from build123d import *

# Parameters (mm, degrees)
SKETCH1_W                    = 41
SKETCH1_H                    = 20
BASE_FLANGE1_DEPTH           = 0.7
EDGE_FLANGE1_STRIP_W         = 4.324
EDGE_FLANGE1_STRIP_H         = 0.7
EDGE_FLANGE1_STRIP_CUT_DEPTH = 20
EDGE_FLANGE1_DEPTH           = 20
EDGE_FLANGE2_STRIP_W         = 4.324
EDGE_FLANGE2_STRIP_H         = 0.7
EDGE_FLANGE2_STRIP_CUT_DEPTH = 20
EDGE_FLANGE2_DEPTH           = 20
M3_CLEARANCE_HOLE1_D         = 3.4


# Sheet-metal steps are written as plain solids
with BuildPart() as part:
    # Sketch1 → Base-Flange1 (new body)
    with BuildSketch(Plane(origin=(0, 0, 0), x_dir=(1, 0, 0), z_dir=(0, 1, 0))):
        with Locations((20.5, 10)):
            Rectangle(SKETCH1_W, SKETCH1_H)
    extrude(amount=-BASE_FLANGE1_DEPTH)

    # Edge-Flange1 strip (across the edge) → Edge-Flange1 strip cut (cut)
    with BuildSketch(Plane(origin=(41, 0, 0), x_dir=(-1, 0, 0), z_dir=(0, 0, -1))):
        with Locations((-1.4, -0.35)):
            Rectangle(EDGE_FLANGE1_STRIP_W, EDGE_FLANGE1_STRIP_H)
    edge_flange1_strip_cut = extrude(amount=EDGE_FLANGE1_STRIP_CUT_DEPTH, mode=Mode.SUBTRACT)

    # Edge-Flange1 section (across the edge) → Edge-Flange1 (add)
    with BuildSketch(Plane(origin=(41, 0, 0), x_dir=(-1, 0, 0), z_dir=(0, 0, -1))):
        with BuildLine():
            Line((-0.7, 0.762), (-0.7, 20.25))
            Line((-0.7, 20.25), (0, 20.25))
            Line((0, 20.25), (0, 0.762))
            ThreePointArc((0, 0.762), (0.223184633, 0.223184633), (0.762, 0))
            Line((0.762, 0), (0.762, -0.7))
            ThreePointArc((0.762, -0.7), (-0.271790114, -0.271790114), (-0.7, 0.762))
        make_face()
    edge_flange1 = extrude(amount=EDGE_FLANGE1_DEPTH)

    # Edge-Flange2 strip (across the edge) → Edge-Flange2 strip cut (cut)
    with BuildSketch(Plane(origin=(41.7, 20.25, -20), x_dir=(0, -1, 0), z_dir=(0, 0, 1))):
        with Locations((-0.7, -0.35)):
            Rectangle(EDGE_FLANGE2_STRIP_W, EDGE_FLANGE2_STRIP_H)
    edge_flange2_strip_cut = extrude(amount=EDGE_FLANGE2_STRIP_CUT_DEPTH, mode=Mode.SUBTRACT)

    # Edge-Flange2 section (across the edge) → Edge-Flange2 (add)
    with BuildSketch(Plane(origin=(41.7, 20.25, -20), x_dir=(0, -1, 0), z_dir=(0, 0, 1))):
        with BuildLine():
            Line((0, 0.762), (0, 15))
            Line((0, 15), (0.7, 15))
            Line((0.7, 15), (0.7, 0.762))
            ThreePointArc((0.7, 0.762), (0.923184633, 0.223184633), (1.462, 0))
            Line((1.462, 0), (1.462, -0.7))
            ThreePointArc((1.462, -0.7), (0.428209886, -0.271790114), (0, 0.762))
        make_face()
    edge_flange2 = extrude(amount=EDGE_FLANGE2_DEPTH)

    # Mirror1: Edge-Flange1 strip cut, Edge-Flange1, Edge-Flange2 strip cut, Edge-Flange2 across plane
    add(edge_flange1_strip_cut.mirror(Plane(origin=(20.5, 0, 0), x_dir=(0, 0, 1), z_dir=(1, 0, 0))), mode=Mode.SUBTRACT)
    add(edge_flange1.mirror(Plane(origin=(20.5, 0, 0), x_dir=(0, 0, 1), z_dir=(1, 0, 0))))
    add(edge_flange2_strip_cut.mirror(Plane(origin=(20.5, 0, 0), x_dir=(0, 0, 1), z_dir=(1, 0, 0))), mode=Mode.SUBTRACT)
    add(edge_flange2.mirror(Plane(origin=(20.5, 0, 0), x_dir=(0, 0, 1), z_dir=(1, 0, 0))))

    # M3 Clearance Hole1 (through all)
    with Locations(Plane(origin=(0, 20.25, 0), x_dir=(1, 0, 0), z_dir=(0, 1, 0))):
        with Locations((49.581, 15), (49.581, 5), (-8.581, 15), (-8.581, 5)):
            Hole(M3_CLEARANCE_HOLE1_D / 2)


solid = part.part
Geometry check sheet. Reference: the model listing, model coordinates, mm. A direction names the side the tool comes from. Round coordinates to 2 decimals unless told otherwise and drop trailing zeros. Write each loop counter-clockwise with the first axis right and the second up, starting at its lowest first coordinate (ties: lowest second). Pieces come first, ordered by that corner, then holes. Notation, with made-up numbers: (10, 43) -> (19, 43) arc R25 cw to (19, 78) -> close; hole circle Ø8 at (16, 82.25). An arc over 180 degrees is marked (long way). One line per item, written item: value. Start each with the question number.
(1) Scan lines: line 1 (X direction, y = 11.5, z = -6.5); line 2 (X direction, y = 19.95, z = -5); line 3 (Y direction, x = 4.5, z = -2.5). Record each from-to range of solid material in increasing order. Write a range as [from, to].
(2) Cross-section at A-A, the plane z = -15. Record the cut outline in (x, y).
(3) Draft check along Y on faces 1 (the cylindrical face through (41.26, -0.283, -9.86)), 2 (the flat face through (20, 0, -10)), 3 (the cylindrical face through (-10.15, 19.9, -14.35)). Enter one of: +Y half, -Y half, draft (parallel to the pull), parting line (faces both ways), or undercut.
(4) Cross-section at C-C, the plane z = -17.75. Record the cut outline in (x, y), and give its area (3 significant figures).
(5) Access from +Z, -Z, +X, -X, +Y, -Y to the whole of each face (thin tool, end or side, straight path). Record for faces 4 (the cylindrical face through (-0.417, 19.81, -10.14)), 5 (the flat face through (-0.7, 10, -10)), 6 (the flat face through (50, 19.55, -10)), 7 (the flat face through (20.3, -0.4, -20)).
(6) Go/stop test with flat-tipped pins: pin 1 Ø4 at (y, z) = (11.5, -6.5) entering from +X; pin 2 Ø2.5 at (x, z) = (-8.581, -15) entering from -Y; pin 3 Ø10 at (x, z) = (17.5, -7.5) entering from +Y; pin 4 Ø4 at (y, z) = (16, -15) entering from -X. Record where each tip stops, or that it passes through.
(7) Cross-section at D-D, the plane x = 20. Record the cut outline in (y, z), and give its area (3 significant figures).
(8) Cross-section at B-B, the plane y = 8. Record the cut outline in (x, z).
Answer:
1. line 1: [-0.7, 0], [41, 41.7]
1. line 2: [-15.7, -10.28], [-6.88, -0.57], [41.57, 47.88], [51.28, 56.7]
1. line 3: [-0.7, 0]
2. outline: (-15.7, 19.55) -> (-10.28, 19.55) -> (-10.28, 20.25) -> (-15.7, 20.25) -> close; (-6.88, 19.55) -> (-1.46, 19.55) arc R0.76 cw to (-0.7, 18.79) -> (-0.7, 0.76) arc R1.46 ccw to (0.76, -0.7) -> (40.24, -0.7) arc R1.46 ccw to (41.7, 0.76) -> (41.7, 18.79) arc R0.76 cw to (42.46, 19.55) -> (47.88, 19.55) -> (47.88, 20.25) -> (42.46, 20.25) arc R1.46 ccw to (41, 18.79) -> (41, 0.76) arc R0.76 cw to (40.24, 0) -> (0.76, 0) arc R0.76 cw to (0, 0.76) -> (0, 18.79) arc R1.46 ccw to (-1.46, 20.25) -> (-6.88, 20.25) -> close; (51.28, 19.55) -> (56.7, 19.55) -> (56.7, 20.25) -> (51.28, 20.25) -> close
3. face 1: -Y half
3. face 2: +Y half
3. face 3: draft
4. outline: (-15.7, 19.55) -> (-1.46, 19.55) arc R0.76 cw to (-0.7, 18.79) -> (-0.7, 0.76) arc R1.46 ccw to (0.76, -0.7) -> (40.24, -0.7) arc R1.46 ccw to (41.7, 0.76) -> (41.7, 18.79) arc R0.76 cw to (42.46, 19.55) -> (56.7, 19.55) -> (56.7, 20.25) -> (42.46, 20.25) arc R1.46 ccw to (41, 18.79) -> (41, 0.76) arc R0.76 cw to (40.24, 0) -> (0.76, 0) arc R0.76 cw to (0, 0.76) -> (0, 18.79) arc R1.46 ccw to (-1.46, 20.25) -> (-15.7, 20.25) -> close
4. area: 77.7 mm²
5. face 4: +Z, -Z, +Y
5. face 5: +Z, -Z, -X, -Y
5. face 6: +Z, -Z, +X, -Y
5. face 7: -Z, +X, -X, +Y, -Y
6. pin 1: x = 41.7
6. pin 2: through
6. pin 3: y = 0
6. pin 4: x = -0.7
7. outline: (-0.7, -20) -> (0, -20) -> (0, 0) -> (-0.7, 0) -> close
7. area: 14.0 mm²
8. outline: (-0.7, -20) -> (0, -20) -> (0, 0) -> (-0.7, 0) -> close; (41, -20) -> (41.7, -20) -> (41.7, 0) -> (41, 0) -> close
